Part print with two shaded views. Sizes in mm from the minimum x, y, z corner. A direction names the side the tool comes from. Round coordinates to 2 decimals unless told otherwise and drop trailing zeros. Order: outer loops, then holes, each group sorted by start corner. A loop starts at its lowest first (then second) coordinate and runs counter-clockwise, first axis right, second up. Notation, with made-up numbers: M -14,-6 L 31,-6 A17 cw 31,25 Z; hole C 14,11.25 d5. An arc over 180 degrees is marked long. Put each result on its own line as item: value.
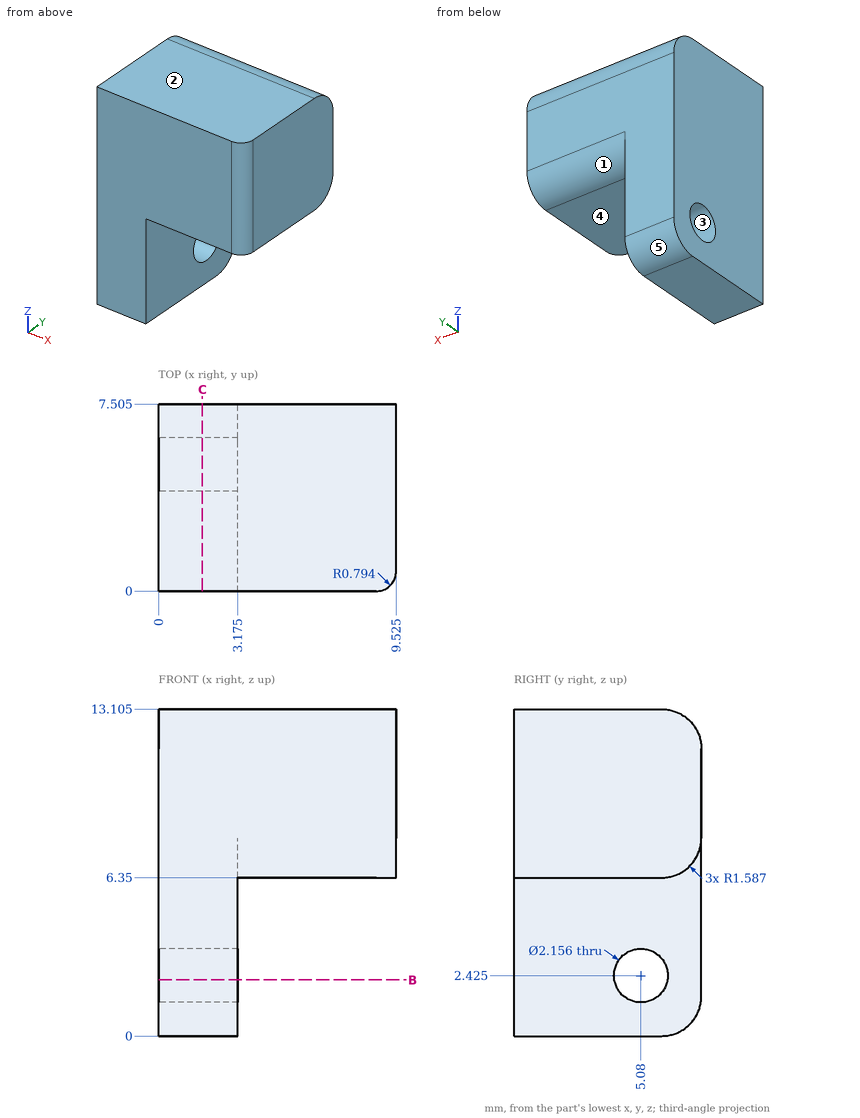
Item 1: Pin check, flat tips, straight feed: P1, Ø2.5, axis at y = 2, z = 5.5, coming from the +X side (1 decimal); P2, Ø1.5, axis at y = 6.5, z = 5, coming from the +X side (1 decimal); P3, Ø3, axis at x = 5.5, y = 3.5, coming from the -Z side. Stop position of each tip, or through.
Answers below:
P1: x = 9.5
P2: x = 3.2
P3: z = 6.35
Item 2: Tool access for the marked faces 4 and 5: list every direction of +Z, -Z, +X, -X, +Y, -Y with a clear straight run to the whole face (end or side of a thin tool).
Answers below:
face 4: -Z, +X, +Y, -Y
face 5: -Z, +X, -X, +Y
Item 3: Band-saw the part on B-B on z = 2.25. Give the cut face in (x, y) (1 decimal).
Answers below:
outline: M 0,0 L 3.2,0 L 3.2,4 L 0,4 Z; M 0,6.1 L 3.2,6.1 L 3.2,7.5 L 0,7.5 Z
Item 4: Mould opens along Y. For the marked faces 1, 2 and 3 say: pulls with the +Y half, pulls with the -Y half, needs draft (parallel to the pull), parting line crosses it, or undercut.
Answers below:
face 1: pulls with the +Y half
face 2: needs draft
face 3: undercut
Item 5: Band-saw the part on C-C on x = 1.75. Give the cut face in (y, z) (1 decimal).
Answers below:
outline: M 0,0 L 5.9,0 A1.6 ccw 7.5,1.6 L 7.5,11.5 A1.6 ccw 5.9,13.1 L 0,13.1 Z; hole C 5.1,2.4 d2.2
Item 6: Probe line 1 along Z through (x, y) = (2.1, 5.08) (1 decimal); line 2 along X through (y, z) = (6.5, 2) (1 decimal); line 3 along Y through (x, z) = (2.25, 3) (1 decimal). List the from-to ranges inside material, lowest first. Write a range as [from, to].
Answers below:
line 1: [0, 1.3], [3.5, 13.1]
line 2: [0, 3.2]
line 3: [0, 4.2], [6, 7.5]
